Autodesk Fusion 360 part; units mm, degrees
sketch "Sketch1" plane through (0, 0, 0) normal (0, 0, 1) x (1, 0, 0)
  line L0 (5, 24) -> (56, 24)
  line L1 (56, 24) -> (56, 16)
  line L2 (56, 16) -> (5, 16)
  line L3 (5, 16) -> (5, 24)
  circle A0 centre (8, 20) radius 1.15
  circle A1 centre (12.5, 20) radius 1.2
  circle A2 centre (17, 20) radius 1.25
  circle A3 centre (21.5, 20) radius 1.3
  circle A4 centre (26.5, 20) radius 1.35
  circle A5 centre (31.5, 20) radius 1.4
  circle A6 centre (36.5, 20) radius 1.45
  circle A7 centre (41.5, 20) radius 1.5
  circle A8 centre (47, 20) radius 1.55
  circle A9 centre (52.5, 20) radius 1.6
  dimension "d1" = 51
  dimension "d2" = 8
  dimension "d6" = 2.3
  dimension "d7" = 2.4
  dimension "d8" = 2.5
  dimension "d9" = 2.6
  dimension "d10" = 2.7
  dimension "d11" = 2.8
  dimension "d12" = 2.9
  dimension "d13" = 3
  dimension "d14" = 3.1
  dimension "d15" = 3.2
extrude "Extrude2" add sketch "Sketch1" along normal blind 5
The listing builds one solid part. Answer for the finished solid, in the listing's coordinates (mm). Coordinates: 2 decimals unless noted, no trailing zeros. Loops run counter-clockwise (first coordinate to the right, second up) from the corner with the lowest first, then second, coordinate; pieces in that order, holes last. Notation, with made-up numbers: (-33, 18.25) -> (15, 18.25) arc R31 ccw to (15, 49.25) -> close; hole circle Ø2 at (84, -8). An arc over 180 degrees is marked (long way). Return JSON: item names as keys, results as strings. Group by question number.
(1) A cutting plane is placed at A-A on x = 47. Write down the section's boundary in (y, z), and give its area (3 significant figures).
(2) Determine the mould class of faces 1 (the flat face through (56, 20, 2)), 2 (the flat face through (5, 20, 2)), 3 (the cylindrical face through (48.478, 19.534, 2.465)), 4 (the flat face through (30, 19, 5)) for opening direction X: released by +X, released by -X, zero draft, split by the parting line, or undercut.
(3) A cutting plane is placed at B-B on z = 1.9. Count the separate pieces of the cut face and the enclosed holes in it, and give its area (3 significant figures).
(4) Find the intervals of material crossed by probe 1 along Y at (x, z) = (27, 0.55); probe 2 along Y at (x, z) = (8, 2), in increasing order. Write a range as from..to.
(5) A cutting plane is placed at C-C on x = 31.5. Write down the section's boundary in (y, z).
(6) Given pin 1 Ø2.5 at (x, y) = (26.5, 20) entering from +Z, flat-ended and moving along its own axis, determine where the tip first touches the part or whether it passes through.
The answers:
{
 "1": {"outline": "(16, 0) -> (18.45, 0) -> (18.45, 5) -> (16, 5) -> close; (21.55, 0) -> (24, 0) -> (24, 5) -> (21.55, 5) -> close", "area": "24.5 mm^2"},
 "2": {"face 1": "released by +X", "face 2": "released by -X", "face 3": "undercut", "face 4": "zero draft"},
 "3": {"separate pieces": "1", "enclosed holes": "10", "area": "348 mm^2"},
 "4": {"probe 1": "y = 16..18.75, 21.25..24", "probe 2": "y = 16..18.85, 21.15..24"},
 "5": {"outline": "(16, 0) -> (18.6, 0) -> (18.6, 5) -> (16, 5) -> close; (21.4, 0) -> (24, 0) -> (24, 5) -> (21.4, 5) -> close"},
 "6": {"pin 1": "passes through"}
}
